Check sheet for the modelled part. Datum: model origin and axes. Units: mm. A direction names the side the tool comes from. Round coordinates to 2 decimals unless told otherwise and drop trailing zeros. Loops run counter-clockwise (first coordinate to the right, second up) from the corner with the lowest first, then second, coordinate; pieces in that order, holes last. Notation, with made-up numbers: (-29.5, 12) - (29.5, 12) arc R30 ccw to (29.5, 50) - close; hole circle Ø10 at (13, 36.5). An arc over 180 degrees is marked (long way). Put each result on its own line as item: value. Start each with the question number.
Item 1: Draft check along X on faces 1 (the cylindrical face through (-26.73, -0.43, 1.48)), 2 (the flat face through (-8.3, 25, 3)), 3 (the flat face through (-25, -1, 0)). Enter one of: pulls with the +X half, pulls with the -X half, needs draft (parallel to the pull), parting line crosses it, or undercut.
Item 2: Material ranges on line 1 along Y through (x, z) = (5, 8.5); line 2 along Y through (x, z) = (-30, 2.1); line 3 along Z through (x, y) = (0, -43.5), recorded low to high.
Item 3: Section check C-C, the plane z = 14.75. Record the cut outline in (x, y), and give its area (3 significant figures).
Item 4: Section check B-B, the plane x = -30. Record the cut outline in (y, z).
Item 5: Tool access check on faces 4 (the conical face through (-26.595, -38.256, 3.188)), 5 (the cylindrical face through (-2.4, -46.9, 4.8)), 6 (the flat face through (-19, -1, 6)), 7 (the cylindrical face through (5.84, -50.18, 13.47)), 8 (the flat face through (-2, 12.5, 4)). Record the directions out of +Z, -Z, +X, -X, +Y, -Y that give a thin tool (end or side, any length) a straight path to the whole face; none if there is none.
Item 6: Gauge pin test, flat ends, axial feed: pin 1 Ø8 at (y, z) = (-35.5, 3) entering from +X; pin 2 Ø2 at (y, z) = (-47.5, 6.5) entering from -X; pin 3 Ø6 at (y, z) = (41.5, 10.5) entering from -X. Record the tip position at first contact, or that the pin passes through.
Item 7: Section check D-D, the plane x = -12. Record the cut outline in (y, z).
Item 8: Section check A-A, the plane y = 0. Record the cut outline in (x, z), and give its area (3 significant figures).
Solid Edge part; units mm, degrees
sketch "Sketch1" plane through (0, 0, 0) normal (0, -1, 0) x (1, 0, 0)
  line L0 (-50, 0) -> (-50, 4)
  arc A0 (-50, 4) -> (-48, 6) centre (-48, 4) cw
  line L1 (-48, 6) -> (-8, 6)
  line L2 (-8, 6) -> (-8, 8)
  arc A1 (-8, 8) -> (0, 0) centre (0, 8) cw
  line L3 (0, 0) -> (-50, 0)
extrude "ExtrudedProtrusion_1" add sketch "Sketch1" against normal blind 62.5 and the other way blind 62.5
sketch "Sketch2" plane through (0, 0, 0) normal (0, 0, 1) x (1, 0, 0)
  line L0 (-8.3, 37.5) -> (-8.3, 12.5)
  line L1 (-8.3, 12.5) -> (16, 12.5)
  line L2 (16, 12.5) -> (16, -12.5)
  line L3 (16, -12.5) -> (-8.3, -12.5)
  line L4 (-8.3, -12.5) -> (-8.3, -37.5)
  line L5 (-8.3, -37.5) -> (21, -37.5)
  line L6 (21, -37.5) -> (21, 37.5)
  line L7 (21, 37.5) -> (-8.3, 37.5)
extrude "ExtrudedCutout_1" cut sketch "Sketch2" along normal blind 16
sketch "Sketch3" plane through (-30, 0, 0) normal (1, 0, 0) x (0, 1, 0)
  line L0 (37.5, 6) -> (43.8, 6)
  line L1 (43.8, 6) -> (40.8, 3)
  line L2 (40.8, 3) -> (40.8, 0)
  line L3 (40.8, 0) -> (37.5, 0)
  line L4 (37.5, 0) -> (37.5, 6)
revolve "RevolvedCutout1" cut sketch "Sketch3" angle 360 about axis through (-30, 37.5, 0) along (0, 0, 1)
sketch "Sketch4" plane through (-30, 0, 0) normal (1, 0, 0) x (0, 1, 0)
  line L0 (-37.5, 6) -> (-31.2, 6)
  line L1 (-31.2, 6) -> (-34.2, 3)
  line L2 (-34.2, 3) -> (-34.2, 0)
  line L3 (-34.2, 0) -> (-37.5, 0)
  line L4 (-37.5, 0) -> (-37.5, 6)
revolve "RevolvedCutout2" cut sketch "Sketch4" angle 360 about axis through (-30, -37.5, 0) along (0, 0, 1)
sketch "Sketch5" plane through (-30, 0, 0) normal (1, 0, 0) x (0, 1, 0)
  line L0 (0, 6) -> (6.3, 6)
  line L1 (6.3, 6) -> (3.3, 3)
  line L2 (3.3, 3) -> (3.3, 0)
  line L3 (3.3, 0) -> (0, 0)
  line L4 (0, 0) -> (0, 6)
revolve "RevolvedCutout3" cut sketch "Sketch5" angle 360 about axis through (-30, 0, 0) along (0, 0, 1)
sketch "Sketch6" plane through (0, 0, 0) normal (1, 0, 0) x (0, 1, 0)
  arc A0 (-60.5, 8) -> (-56.5, 12) centre (-56.5, 8) cw
  line L0 (-56.5, 12) -> (56.5, 12)
  arc A1 (56.5, 12) -> (60.5, 8) centre (56.5, 8) cw
  line L1 (60.5, 8) -> (-60.5, 8)
revolve "RevolvedCutout4" cut sketch "Sketch6" angle 360 about axis through (0, 60.5, 8) along (0, -1, 0)
Check result:
1. face 1: undercut
1. face 2: pulls with the +X half
1. face 3: needs draft
2. line 1: -62.5 to -37.5, -12.5 to 12.5, 37.5 to 62.5
2. line 2: -62.5 to -40.8, -34.2 to -3.3, 3.3 to 34.2, 40.8 to 62.5
2. line 3: 0 to 4, 12 to 16
3. outline: (-4.29, -62.5) - (4.29, -62.5) - (4.29, -37.5) - (-4.29, -37.5) - close; (-4.29, -12.5) - (4.29, -12.5) - (4.29, 12.5) - (-4.29, 12.5) - close; (-4.29, 37.5) - (4.29, 37.5) - (4.29, 62.5) - (-4.29, 62.5) - close
3. area: 644 mm²
4. outline: (-62.5, 0) - (-40.8, 0) - (-40.8, 3) - (-43.8, 6) - (-62.5, 6) - close; (-34.2, 0) - (-3.3, 0) - (-3.3, 3) - (-6.3, 6) - (-31.2, 6) - (-34.2, 3) - close; (3.3, 0) - (34.2, 0) - (34.2, 3) - (31.2, 6) - (6.3, 6) - (3.3, 3) - close; (40.8, 0) - (62.5, 0) - (62.5, 6) - (43.8, 6) - (40.8, 3) - close
5. face 4: +Z
5. face 5: none
5. face 6: +Z, -X, +Y, -Y
5. face 7: +Y, -Y
5. face 8: +Z, -Z, +X
6. pin 1: x = 7.85
6. pin 2: x = -49.32
6. pin 3: x = -8
7. outline: (-62.5, 0) - (62.5, 0) - (62.5, 6) - (-62.5, 6) - close
8. outline: (-50, 0) - (-33.3, 0) - (-33.3, 3) - (-36.3, 6) - (-48, 6) arc R2 ccw to (-50, 4) - close; (-26.7, 0) - (0, 0) arc R8 ccw (long way) to (-8, 8) - (-8, 6) - (-23.7, 6) - (-26.7, 3) - close; hole circle Ø8 at (0, 8)
8. area: 367 mm²
